Verification items for the finished model (mm, model axes). Face numbers are marked on the shaded views. Round coordinates to 2 decimals unless told otherwise and drop trailing zeros. Order: outer loops, then holes, each group sorted by start corner. A loop starts at its lowest first (then second) coordinate and runs counter-clockwise, first axis right, second up.
```python
from build123d import *
from OCP.BRepFilletAPI import BRepFilletAPI_MakeChamfer

# Parameters (mm, degrees)
SALIENTE_EXTRUIR1_DEPTH = 6
CHAFL_N1_SIZE           = 6
CHAFL_N1_SIZE2          = 1.607695155
CORTAR_EXTRUIR1_DEPTH   = 3
SALIENTE_EXTRUIR2_DEPTH = 15
CORTAR_EXTRUIR5_START   = -13
CORTAR_EXTRUIR5_DEPTH   = 26
CORTAR_EXTRUIR6_DEPTH   = 92.438482365
CORTAR_EXTRUIR7_START   = -13
CORTAR_EXTRUIR7_DEPTH   = 26
CROQUIS12_R             = 4.5
CORTAR_EXTRUIR8_DEPTH   = 3
CROQUIS13_R             = 1
CORTAR_EXTRUIR9_DEPTH   = 93.238012844


# Read off the part's stored shape, not the designer's step: Cortar-Extruir5, Cortar-Extruir7
with BuildPart() as part:
    # Croquis1 → Saliente-Extruir1 (new body)
    with BuildSketch(Plane.XY):
        Polygon((0, 11), (-90, 11), (-90, -11), (0, -11), (42, -13), (42, 13), align=None)
    extrude(amount=SALIENTE_EXTRUIR1_DEPTH)

    # Chaflán1: one chamfer whose edges measure the first distance from different faces: ONE call of the kernel's chamfer builder (chamfer() names one face for all edges)
    chafl_n1_edges_1 = [part.edges().sort_by_distance(p)[0] for p in [
        (-90, 11, 3),
    ]]
    chafl_n1_side_1 = [part.faces().sort_by_distance(p)[0] for p in [
        (-45, 11, 3),
    ]]
    chafl_n1_edges_2 = [part.edges().sort_by_distance(p)[0] for p in [
        (-90, -11, 3),
    ]]
    chafl_n1_side_2 = [part.faces().sort_by_distance(p)[0] for p in [
        (-45, -11, 3),
    ]]
    chafl_n1 = BRepFilletAPI_MakeChamfer(part.part.solid().wrapped)
    for e in chafl_n1_edges_1:
        chafl_n1.Add(CHAFL_N1_SIZE, CHAFL_N1_SIZE2, e.wrapped, chafl_n1_side_1[0].wrapped)  # the first distance lies on this face
    for e in chafl_n1_edges_2:
        chafl_n1.Add(CHAFL_N1_SIZE, CHAFL_N1_SIZE2, e.wrapped, chafl_n1_side_2[0].wrapped)  # the first distance lies on this face
    add(Compound.cast(chafl_n1.Shape()), mode=Mode.REPLACE)

    # Croquis7 → Cortar-Extruir1 (cut)
    with BuildSketch(Plane.XY.offset(6)):
        Polygon((-88, 7.857650869), (-88, -7.857650869), (-83.736695005, -9), (0.047592083, -9), (42, -10.99773371), (42, -6), (-86, -6), (-86, -4), (42, -4), (42, 4), (-86, 4), (-86, 6), (42, 6), (42, 10.99773371), (0.047592083, 9), (-83.736695005, 9), align=None)
    extrude(amount=-CORTAR_EXTRUIR1_DEPTH, mode=Mode.SUBTRACT)

    # Croquis3 → Saliente-Extruir2 (add, symmetric)
    with BuildSketch(Plane(origin=(-88, 0, 0), x_dir=(0, 0, 1), z_dir=(0, -1, 0))):
        with BuildLine():
            Line((4, -13), (4, -88))
            Line((4, -88), (5, -127))
            Line((5, -127), (5, -130))
            Line((5, -130), (0, -130))
            Line((0, -130), (0, 2))
            Line((0, 2), (3, 2))
            ThreePointArc((3, 2), (3.129320027, 1.000556782), (3.249721603, 0))
            ThreePointArc((3.249721603, 0), (3.812274468, -6.48918366), (4, -13))
        make_face()
    extrude(amount=SALIENTE_EXTRUIR2_DEPTH, both=True)

    # Cortar-Extruir5 outline → Cortar-Extruir5 (cut)
    with BuildSketch(Plane(origin=(0, 0, 0), x_dir=(1, 0, 0), z_dir=(0, 1, 0)).offset(CORTAR_EXTRUIR5_START)):
        with BuildLine():
            Line((-0.012818406, -5), (-75, -5))
            ThreePointArc((-75, -5), (-80.506427226, -4.866936638), (-86, -4.468057179))
            ThreePointArc((-86, -4.468057179), (-88.002027457, -4.256113663), (-90, -4.008849211))
            Line((-90, -4.008849211), (-90, -6))
            Line((-90, -6), (42, -6))
            Line((42, -6), (42, -5.999671431))
            Line((42, -5.999671431), (38.974367399, -5.999671431))
            Line((38.974367399, -5.999671431), (-0.012818406, -5))
        make_face()
    extrude(amount=CORTAR_EXTRUIR5_DEPTH, mode=Mode.SUBTRACT)

    # Croquis9 → Cortar-Extruir6 (cut, through all)
    with BuildSketch(Plane(origin=(0, 0, 0), x_dir=(-1, 0, 0), z_dir=(0, 0, -1))):
        Polygon((-39, 12.857142857), (0, 11), (75, 11), (84, 11), (90, 9.392304845), (90, 15), (-42, 15), (-42, 13), align=None)
        Polygon((-39, -12.857142857), (-42, -13), (-42, -15), (90, -15), (90, -9.392304845), (84, -11), (75, -11), (0, -11), align=None)
    extrude(amount=-CORTAR_EXTRUIR6_DEPTH, mode=Mode.SUBTRACT)

    # Cortar-Extruir7 outline → Cortar-Extruir7 (cut)
    with BuildSketch(Plane(origin=(0, 0, 0), x_dir=(1, 0, 0), z_dir=(0, 1, 0)).offset(CORTAR_EXTRUIR7_START)):
        with BuildLine():
            Line((42, -5.999671431), (42, -2.999890938))
            ThreePointArc((42, -2.999890938), (41.130433899, -5.112013503), (39.025850725, -5.999671431))
            Line((39.025850725, -5.999671431), (42, -5.999671431))
        make_face()
        with BuildLine():
            ThreePointArc((39.000109062, 0), (41.121352287, -0.878647713), (42, -2.999890938))
            Line((42, -2.999890938), (42, 0))
            Line((42, 0), (39.000109062, 0))
        make_face()
    extrude(amount=CORTAR_EXTRUIR7_DEPTH, mode=Mode.SUBTRACT)

    # Croquis12 → Cortar-Extruir8 (cut)
    with BuildSketch(Plane(origin=(-0.522624434, -10.975113122, 0), x_dir=(0.9988681377244376, -0.04756514941544958, 0), z_dir=(-0.04756514941544957, -0.9988681377244375, 0))):
        with Locations((39.567518478, 2.999890938)):
            Circle(CROQUIS12_R)
    cortar_extruir8 = extrude(amount=-CORTAR_EXTRUIR8_DEPTH, mode=Mode.SUBTRACT)

    # Croquis13 → Cortar-Extruir9 (cut, through all)
    with BuildSketch(Plane(origin=(-0.379928986, -7.978508709, 0), x_dir=(0.9988681377244376, -0.0475651494154496, 0), z_dir=(-0.04756514941544959, -0.9988681377244375, 0))):
        with Locations((39.567518478, 2.999890938)):
            Circle(CROQUIS13_R)
    extrude(amount=-CORTAR_EXTRUIR9_DEPTH, mode=Mode.SUBTRACT)

    # Simetría1: Cortar-Extruir8 across plane
    add(cortar_extruir8.mirror(Plane.ZX), mode=Mode.SUBTRACT)


solid = part.part
```
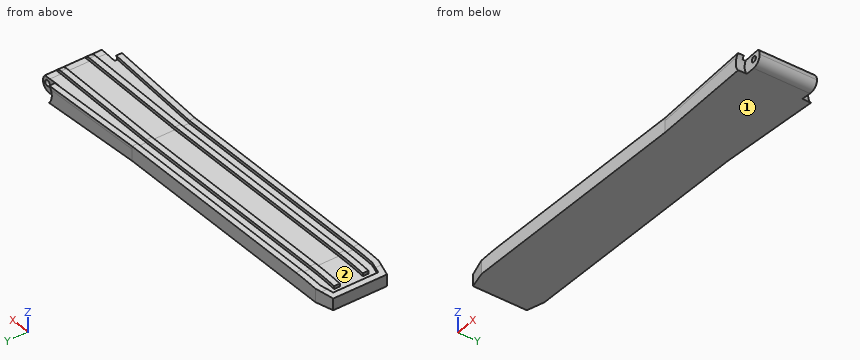
1) Scan lines: probe 1 along Y at (x, z) = (-70, 4.85); probe 2 along Y at (x, z) = (26.5, 5.5); probe 3 along Z at (x, y) = (-77, -3.5). Record each from-to range of solid material in increasing order.
2) Go/stop test with flat-tipped pins: pin 1 Ø1 at (x, z) = (-25, 3.5) entering from +Y; pin 2 Ø2 at (y, z) = (7.5, 1) entering from +X; pin 3 Ø1.6 at (x, y) = (-44, -10) entering from +Z. Record where each tip stops, or that it passes through.
3) Sectioned sample at A-A on x = -47. Record the cut outline in (y, z).
4) Draft check along Y on the marked faces 1 and 2. Enter one of: released by +Y, released by -Y, zero draft, split by the parting line, or undercut.
5) Sectioned sample at B-B on x = -78. Record the cut outline in (y, z), then the cut area to 3 significant figures.
Returned:
1. probe 1: y = -11 to -9, -6 to -4, 4 to 6, 9 to 11
1. probe 2: y = -12.26 to -10.26, -6 to -4, 4 to 6, 10.26 to 12.26
1. probe 3: z = 0 to 3.98
2. pin 1: stops at y = 11
2. pin 2: stops at x = 41.83
2. pin 3: stops at z = 5
3. outline: (-11, 0) - (11, 0) - (11, 5) - (9, 5) - (9, 4) - (6, 4) - (6, 5) - (4, 5) - (4, 4) - (-4, 4) - (-4, 5) - (-6, 5) - (-6, 4) - (-9, 4) - (-9, 5) - (-11, 5) - close
4. face 1: zero draft
4. face 2: undercut
5. outline: (-11, 0) - (11, 0) - (11, 4.96) - (9, 4.96) - (9, 3.96) - (6, 3.96) - (6, 4.96) - (4, 4.96) - (4, 3.96) - (-4, 3.96) - (-4, 4.96) - (-6, 4.96) - (-6, 3.96) - (-9, 3.96) - (-9, 4.96) - (-11, 4.96) - close
5. area: 95.1 mm2
